CAD build for the part. Positions are in the model's coordinates, mm. A direction names the side the tool comes from. Round coordinates to 2 decimals unless told otherwise and drop trailing zeros. Order: outer loops, then holes, each group sorted by start corner. A loop starts at its lowest first (then second) coordinate and runs counter-clockwise, first axis right, second up. Notation, with made-up numbers: M 54.25,14.5 L 92.25,14.5 A18 ccw 92.25,22.5 Z; hole C -22.75,-28.5 d3. An arc over 180 degrees is marked long. Answer as a JSON object with one key per item and string values.
```python
from build123d import *

# Parameters (mm, degrees)
F2_DEPTH = 385
F1_R     = 2.75
F3_DEPTH = 2.75


with BuildPart() as f2:
    # F0 (on Front) → F2 (new body)
    with BuildSketch(Plane.XZ):
        with BuildLine():
            Line((20, -2.5), (20, 2.5))
            Line((20, 2.5), (3, 2.5))
            Line((3, 2.5), (3, 15.0838015129))
            ThreePointArc((3, 15.0838015129), (0, 30.5), (-3, 15.0838015129))
            Line((-3, 15.0838015129), (-3, 2.5))
            Line((-3, 2.5), (-20, 2.5))
            Line((-20, 2.5), (-20, -2.5))
            Line((-20, -2.5), (20, -2.5))
        make_face()
    extrude(amount=-F2_DEPTH)

    # F1 (on Top) → F3 (cut, symmetric)
    with BuildSketch(Plane.XY):
        with Locations((15, 50)):
            Circle(F1_R)
        with Locations((15, 200)):
            Circle(F1_R)
        with Locations((15, 350)):
            Circle(F1_R)
        with Locations((-15, 50)):
            Circle(F1_R)
        with Locations((-15, 200)):
            Circle(F1_R)
        with Locations((-15, 350)):
            Circle(F1_R)
    extrude(amount=F3_DEPTH, both=True, mode=Mode.SUBTRACT)


solid = f2.part
```
Item 1: Saw through at A-A on y = 65.5. List the corners of the cut face in (x, z).
Worked answers:
{"outline": "M -20,-2.5 L 20,-2.5 L 20,2.5 L 3,2.5 L 3,15.08 A8 ccw long -3,15.08 L -3,2.5 L -20,2.5 Z"}
Item 2: Two-plate mould, pull along Z, no slides. Class faces 4 (the flat face through (-3, 190, 9)), 5 (the flat face through (0, 385, 12)), 6 (the flat face through (0, 190, -2.5)): released by +Z, released by -Z, zero draft, split by the parting line, or undercut.
Worked answers:
{"face 4": "undercut", "face 5": "zero draft", "face 6": "released by -Z"}
Item 3: Drop flat-ended pins along their axis: pin 1 Ø5 at (x, y) = (-15, 350) entering from -Z; pin 2 Ø9 at (x, y) = (-15, 200) entering from +Z; pin 3 Ø18.5 at (x, y) = (12.5, 151) entering from +Z; pin 4 Ø4 at (y, z) = (187, 7) entering from +X. Give the stop position or say it passes through.
Worked answers:
{"pin 1": "passes through", "pin 2": "stops at z = 2.5", "pin 3": "stops at z = 29.81", "pin 4": "stops at x = 3"}
Item 4: Saw through at B-B on z = 22.5. List the corners of the cut face in (x, y).
Worked answers:
{"outline": "M -8,0 L 8,0 L 8,385 L -8,385 Z"}
Item 5: Saw through at C-C on z = 8.5. List the corners of the cut face in (x, y), and give its area (3 significant figures).
Worked answers:
{"outline": "M -3,0 L 3,0 L 3,385 L -3,385 Z", "area": "2,310 mm2"}
Item 6: Wall check: line 1 along X through (y, z) = (200, 1); line 2 along Y through (x, z) = (-15, 0.8); line 3 along Y through (x, z) = (13.5, 1). Give the ranges that are in metal, low to high. Write a range as [from, to].
Worked answers:
{"line 1": "x = [-20, -17.75], [-12.25, 12.25], [17.75, 20]", "line 2": "y = [0, 47.25], [52.75, 197.25], [202.75, 347.25], [352.75, 385]", "line 3": "y = [0, 47.7], [52.3, 197.7], [202.3, 347.7], [352.3, 385]"}
Item 7: 3-axis set-ups, long thin cutter, end or side, ignore diameter. For faces 1 (the flat face through (0, 0, 12)), 2 (the flat face through (-11, 190, 2.5)), 3 (the flat face through (12, 190, 2.5)): which of +Z, -Z, +X, -X, +Y, -Y reach the whole face in a straight line?
Worked answers:
{"face 1": "+Z, -Z, +X, -X, -Y", "face 2": "-X, +Y, -Y", "face 3": "+X, +Y, -Y"}
